Here's the drawing with two shaded views (mm, measured from the low corner). I have some questions. A direction names the side the tool comes from. Give positions to 0.01 mm unless a question says otherwise; leave off trailing zeros. Loops run counter-clockwise (first coordinate to the right, second up) from the corner with the lowest first, then second, coordinate; pieces in that order, holes last. Notation, with made-up numbers: M -10.5,-33 L 17.5,-33 A9 cw 17.5,-26 Z; hole C 12,0 d11. An arc over 180 degrees is marked long. Use CSV: the item, a comma, the result in double quotes.
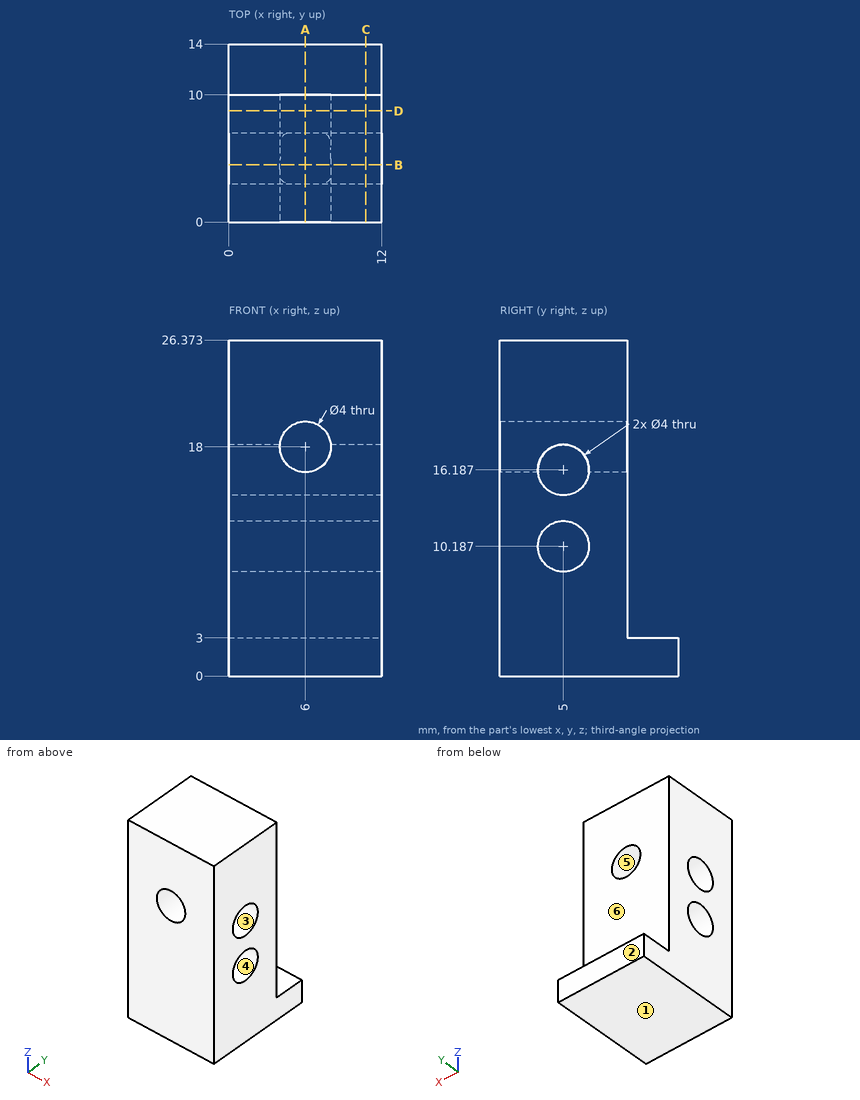
1. I want a section at C-C, the plane x = 10.75. List the corners of the cut face in (y, z) for me.
Outcome:
outline,"M 0,0 L 14,0 L 14,3 L 10,3 L 10,26.37 L 0,26.37 Z; hole C 5,10.19 d4; hole C 5,16.19 d4"
2. I want a section at A-A, the plane x = 6. List the corners of the cut face in (y, z) for me, then the cut area to 3 significant figures.
Outcome:
outline,"M 0,0 L 14,0 L 14,3 L 10,3 L 10,16 L 6.99,16 A2 cw 3.01,16 L 0,16 Z; M 0,20 L 10,20 L 10,26.37 L 0,26.37 Z; hole C 5,10.19 d4"
area,"218 mm2"
3. I'm going to push flat-ended pins straight in: pin 1 Ø3.5 at (x, z) = (9, 17) entering from +Y; pin 2 Ø2 at (x, y) = (3.5, 12.5) entering from +Z. Where does each tip first touch, or does it pass through?
Outcome:
pin 1,"y = 10"
pin 2,"z = 3"
4. I want a section at B-B, the plane y = 4.5. List the corners of the cut face in (x, z) for me.
Outcome:
outline,"M 0,0 L 12,0 L 12,8.25 L 0,8.25 Z; M 0,12.12 L 12,12.12 L 12,14.25 L 0,14.25 Z; M 0,18.12 L 4,18.12 A2 cw 8,18.12 L 12,18.12 L 12,26.37 L 0,26.37 Z"
5. If we mould it in two halves opening along Y, with no side actions, what happens to the marked faces 1, 2, 3 and 4? For each: +Y half, -Y half, draft (parallel to the pull), parting line (faces both ways), or undercut.
Outcome:
face 1,"draft"
face 2,"+Y half"
face 3,"undercut"
face 4,"undercut"
6. Please list where these lines run through material, in increasing order: line 1 (X direction, y = 6.5, z = 18); line 2 (Z direction, x = 8.75, y = 3.5) (1 decimal); line 3 (Y direction, x = 11, z = 20).
Outcome:
line 1,"0 to 4, 8 to 12"
line 2,"0 to 8.9, 11.5 to 14.9, 17.5 to 26.4"
line 3,"0 to 10"
7. I want a section at D-D, the plane y = 8.75. List the corners of the cut face in (x, z) for me, then the cut area to 3 significant figures.
Outcome:
outline,"M 0,0 L 12,0 L 12,26.37 L 0,26.37 Z; hole C 6,18 d4"
area,"304 mm2"
8. Which directions (+Z, -Z, +X, -X, +Y, -Y) give clear straight access to the entire face, cutting with the end or side of a thin tool? Please do the marked faces 5 and 6.
Outcome:
face 5,"+Y, -Y"
face 6,"+Z, +X, -X, +Y"
